Part model, mm, in its own coordinate system. Face numbers are marked on the shaded views. A direction names the side the tool comes from. Give positions to 0.01 mm unless a question says otherwise; leave off trailing zeros. Write each loop counter-clockwise with the first axis right and the second up, starting at its lowest first coordinate (ties: lowest second). Pieces come first, ordered by that corner, then holes. Notation, with made-up numbers: M 26.25,-24 L 84.25,-24 A22 cw 84.25,12 Z; hole C 76.5,89 d3. An arc over 180 degrees is marked long. Answer as CSV lines item,"result". Start each with the question number.
1) Slice it at D-D, the plane z = 60.5. Give the cut face in (x, y), plus the area to 3 significant figures.
2) Tool access for the marked faces 4, 5 and 6: list every direction of +Z, -Z, +X, -X, +Y, -Y with a clear straight run to the whole face (end or side of a thin tool).
3) Wall check: line 1 along Z through (x, y) = (3.25, -0.25); line 2 along X through (y, z) = (1.75, 24.5); line 3 along Z through (x, y) = (11.25, 4). Give the ranges that are in metal, low to high. Write a range as from..to.
4) Slice it at B-B, the plane z = 44. Give the cut face in (x, y).
5) Slice it at A-A, the plane y = 8. Give the cut face in (x, z).
6) Slice it at C-C, the plane x = 0. Give the cut face in (y, z), plus the area to 3 significant figures.
7) Mould opens along X. For the marked faces 1, 2 and 3 say: pulls with the +X half, pulls with the -X half, needs draft (parallel to the pull), parting line crosses it, or undercut.
8) Pin check, flat tips, straight feed: pin 1 Ø0.6 at (x, y) = (3, -0.5) entering from +Z; pin 2 Ø6 at (x, y) = (-3, 8.5) entering from -Z; pin 3 Ø11 at (x, z) = (1.5, 7.5) entering from +Y; pin 4 Ø2.5 at (y, z) = (4, 60.5) entering from +X. Stop position of each tip, or through.
```python
from build123d import *

# Parameters (mm, degrees)
SKETCH_R        = 2
SKETCH_R_2      = 3
PAD_DEPTH       = 2
SKETCH001_W     = 2.1
SKETCH001_H     = 20
PAD001_DEPTH    = 9
CHAMFER_SIZE    = 3
SKETCH002_W     = 13
SKETCH002_H     = 25
POCKET_DEPTH    = 2.5
SKETCH003_R     = 3.5
PAD002_DEPTH    = 1.5
SKETCH004_R     = 1.7
POCKET001_DEPTH = 3
CHAMFER001_SIZE = 0.2
CHAMFER002_SIZE = 0.3
SKETCH005_W     = 3
SKETCH005_H     = 15
PAD003_DEPTH    = 10
CHAMFER003_SIZE = 3
CHAMFER004_SIZE = 3
SKETCH006_W     = 2.1
SKETCH006_H     = 30
PAD004_DEPTH    = 3
SKETCH007_W     = 26.5
SKETCH007_H     = 12
PAD005_DEPTH    = 10
CHAMFER005_SIZE = 2
CHAMFER006_SIZE = 2
CHAMFER007_SIZE = 2
SKETCH008_W     = 10
SKETCH008_H     = 12
POCKET002_DEPTH = 9
SKETCH009_R     = 1.5
POCKET003_DEPTH = 26.501
SKETCH010_R     = 2.75
POCKET004_DEPTH = 1.7


with BuildPart() as part:
    # Sketch → Pad (new body)
    with BuildSketch(Plane.XZ):
        Polygon((-13.25, 55), (13.25, 55), (13.25, -10), (-13.25, -10), (-13.25, -3.15), (-5.5, -3.15), (-5.5, 0), (-5.5, 3.15), (-13.25, 3.15), align=None)
        with Locations((-8.5, 20)):
            Circle(SKETCH_R, mode=Mode.SUBTRACT)
        with Locations((8.5, 20)):
            Circle(SKETCH_R, mode=Mode.SUBTRACT)
        Circle(SKETCH_R_2, mode=Mode.SUBTRACT)
    extrude(amount=PAD_DEPTH)

    # Sketch001 (on Face13 of Pad) → Pad001 (join)
    with BuildSketch(Plane(origin=(0, 0, 0), x_dir=(1, 0, 0), z_dir=(0, 1, 0))):
        with Locations((-12.2, 0)):
            Rectangle(SKETCH001_W, SKETCH001_H)
        with Locations((12.2, 0)):
            Rectangle(SKETCH001_W, SKETCH001_H)
    extrude(amount=PAD001_DEPTH)

    # Chamfer
    chamfer_edges = [part.edges().sort_by_distance(p)[0] for p in [
        (-12.2, 9, -10),
        (12.2, 9, -10),
        (12.2, 9, 10),
        (-12.2, 9, 10),
    ]]
    chamfer(chamfer_edges, length=CHAMFER_SIZE)

    # Sketch002 (on Face4 of Chamfer) → Pocket (cut)
    with BuildSketch(Plane(origin=(0, 0, 0), x_dir=(1, 0, 0), z_dir=(0, 1, 0))):
        with Locations((0, -39.5)):
            Rectangle(SKETCH002_W, SKETCH002_H)
    extrude(amount=-POCKET_DEPTH, mode=Mode.SUBTRACT)

    # Sketch003 (on Face9 of Pocket) → Pad002 (join)
    with BuildSketch(Plane(origin=(-13.25, 0, 0), x_dir=(0, 0, -1), z_dir=(-1, 0, 0))):
        with Locations((0, -3.5)):
            Circle(SKETCH003_R)
    extrude(amount=PAD002_DEPTH)

    # Sketch004 (on Face35 of Pad002) → Pocket001 (cut)
    with BuildSketch(Plane(origin=(-14.75, 0, 0), x_dir=(0, 0, -1), z_dir=(-1, 0, 0))):
        with Locations((0, -3.5)):
            Circle(SKETCH004_R)
    extrude(amount=-POCKET001_DEPTH, mode=Mode.SUBTRACT)

    # Chamfer001
    chamfer001_edges = [part.edges().sort_by_distance(p)[0] for p in [
        (-14.75, 3.5, 1.7),
    ]]
    chamfer(chamfer001_edges, length=CHAMFER001_SIZE)

    # Chamfer002
    chamfer002_edges = [part.edges().sort_by_distance(p)[0] for p in [
        (-14.75, 3.5, 3.5),
    ]]
    chamfer(chamfer002_edges, length=CHAMFER002_SIZE)

    # Sketch005 (on Face17 of Chamfer002) → Pad003 (join)
    with BuildSketch(Plane(origin=(0, 0, 0), x_dir=(1, 0, 0), z_dir=(0, 1, 0))):
        with Locations((-11.75, -47.5)):
            Rectangle(SKETCH005_W, SKETCH005_H)
        with Locations((11.75, -47.5)):
            Rectangle(SKETCH005_W, SKETCH005_H)
    extrude(amount=PAD003_DEPTH)

    # Chamfer003
    chamfer003_edges = [part.edges().sort_by_distance(p)[0] for p in [
        (11.75, 10, 40),
    ]]
    chamfer(chamfer003_edges, length=CHAMFER003_SIZE)

    # Chamfer004
    chamfer004_edges = [part.edges().sort_by_distance(p)[0] for p in [
        (-11.75, 10, 40),
    ]]
    chamfer(chamfer004_edges, length=CHAMFER004_SIZE)

    # Sketch006 (on Face4 of Chamfer004) → Pad004 (join)
    with BuildSketch(Plane(origin=(0, 0, 0), x_dir=(1, 0, 0), z_dir=(0, 1, 0))):
        with Locations((-12.2, -25)):
            Rectangle(SKETCH006_W, SKETCH006_H)
        with Locations((12.2, -25)):
            Rectangle(SKETCH006_W, SKETCH006_H)
    extrude(amount=PAD004_DEPTH)

    # Sketch007 (on Face17 of Pad004) → Pad005 (join)
    with BuildSketch(Plane(origin=(0, 0, 55), x_dir=(-1, 0, 0), z_dir=(0, 0, 1))):
        with Locations((0, -4)):
            Rectangle(SKETCH007_W, SKETCH007_H)
    extrude(amount=PAD005_DEPTH)

    # Chamfer005
    chamfer005_edges = [part.edges().sort_by_distance(p)[0] for p in [
        (-10.25, 5, 55),
    ]]
    chamfer(chamfer005_edges, length=CHAMFER005_SIZE)

    # Chamfer006
    chamfer006_edges = [part.edges().sort_by_distance(p)[0] for p in [
        (10.25, 5, 55),
    ]]
    chamfer(chamfer006_edges, length=CHAMFER006_SIZE)

    # Chamfer007
    chamfer007_edges = [part.edges().sort_by_distance(p)[0] for p in [
        (0, 0, 55),
    ]]
    chamfer(chamfer007_edges, length=CHAMFER007_SIZE)

    # Sketch008 (on Face57 of Chamfer007) → Pocket002 (cut)
    with BuildSketch(Plane(origin=(0, 0, 65), x_dir=(-1, 0, 0), z_dir=(0, 0, 1))):
        with Locations((0, -4)):
            Rectangle(SKETCH008_W, SKETCH008_H)
    extrude(amount=-POCKET002_DEPTH, mode=Mode.SUBTRACT)

    # Sketch009 (on Face51 of Pocket002) → Pocket003 (cut, through all)
    with BuildSketch(Plane(origin=(-13.25, 0, 0), x_dir=(0, 0, -1), z_dir=(-1, 0, 0))):
        with Locations((-60.5, -4)):
            Circle(SKETCH009_R)
    extrude(amount=-POCKET003_DEPTH, mode=Mode.SUBTRACT)

    # Sketch010 (on Face51 of Pocket003) → Pocket004 (cut)
    with BuildSketch(Plane(origin=(-13.25, 0, 0), x_dir=(0, 0, -1), z_dir=(-1, 0, 0))):
        with Locations((-60.5, -4)):
            Circle(SKETCH010_R)
    extrude(amount=-POCKET004_DEPTH, mode=Mode.SUBTRACT)


solid = part.part
```
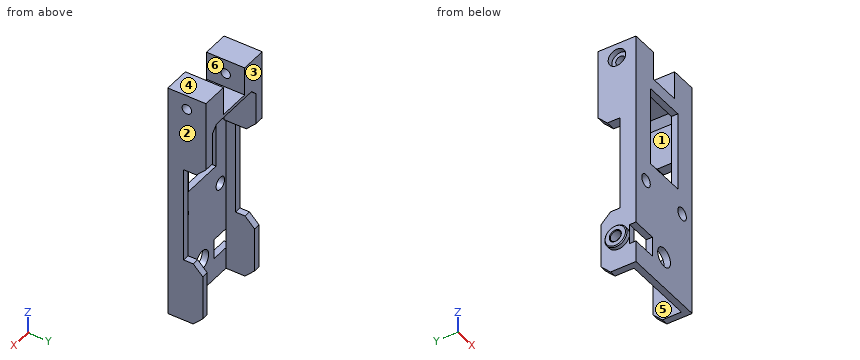
Found:
1,outline,"M -13.25,-2 L -5,-2 L -5,2.5 L -11.55,2.5 L -11.55,1.25 L -13.25,1.25 Z; M -13.25,6.75 L -11.55,6.75 L -11.55,5.5 L -5,5.5 L -5,10 L -13.25,10 Z; M 5,-2 L 13.25,-2 L 13.25,2.5 L 5,2.5 Z; M 5,5.5 L 13.25,5.5 L 13.25,10 L 5,10 Z"
1,area,"144 mm²"
2,face 4,"+Z, +X, -X, +Y, -Y"
2,face 5,"-Z, +Y"
2,face 6,"+Z, +Y, -Y"
3,line 1,"-10..27, 52..56"
3,line 2,"-13.25..-11.15, 11.15..13.25"
3,line 3,"-10..10, 40..59, 62..65"
4,outline,"M -13.25,-2 L -6.5,-2 L -6.5,0 L -10.25,0 L -10.25,10 L -13.25,10 Z; M 6.5,-2 L 13.25,-2 L 13.25,10 L 10.25,10 L 10.25,0 L 6.5,0 Z"
5,outline,"M -13.25,-8 L -11.15,-8 L -11.15,8 L -13.25,8 Z; M -13.25,41 L -10.25,41 L -10.25,53 L -8.25,55 L 8.25,55 L 10.25,53 L 10.25,41 L 13.25,41 L 13.25,65 L 5,65 L 5,56 L -5,56 L -5,65 L -13.25,65 Z; M 11.15,-8 L 13.25,-8 L 13.25,8 L 11.15,8 Z"
6,outline,"M -2,-10 L 0,-10 L 0,-3 L -2,-3 Z; M -2,3 L 0,3 L 0,27 L -2,27 Z; M -2,52 L 0,52 L 0,53 L 2,55 L 10,55 L 10,56 L -2,56 Z"
6,area,"82.0 mm²"
7,face 1,"undercut"
7,face 2,"pulls with the +X half"
7,face 3,"needs draft"
8,pin 1,"z = 56"
8,pin 2,"z = 55"
8,pin 3,"y = 0"
8,pin 4,"through"
